```python
from build123d import *

# Parameters (mm, degrees)
SKETCH1_W               = 36
SKETCH1_H               = 36
SKETCH1_R               = 2.15
BOSS_EXTRUDE1_DEPTH     = 3
BOSS_EXTRUDE2_START     = 2
BOSS_EXTRUDE2_OUTLINE_W = 36
BOSS_EXTRUDE2_OUTLINE_H = 36
BOSS_EXTRUDE2_DEPTH     = 2


# Read off the part's stored shape, not the designer's step: Boss-Extrude2
with BuildPart() as part:
    # Sketch1 → Boss-Extrude1 (new, symmetric)
    with BuildSketch(Plane.XY):
        Rectangle(SKETCH1_W, SKETCH1_H)
        with Locations((-15.5, 15.5)):
            Circle(SKETCH1_R, mode=Mode.SUBTRACT)
        with Locations((15.5, 15.5)):
            Circle(SKETCH1_R, mode=Mode.SUBTRACT)
        with Locations((15.5, -15.5)):
            Circle(SKETCH1_R, mode=Mode.SUBTRACT)
        with Locations((-15.5, -15.5)):
            Circle(SKETCH1_R, mode=Mode.SUBTRACT)
    extrude(amount=BOSS_EXTRUDE1_DEPTH, both=True)

    # Boss-Extrude2 outline → Boss-Extrude2 (add)
    with BuildSketch(Plane.XY.offset(BOSS_EXTRUDE2_START)):
        Rectangle(BOSS_EXTRUDE2_OUTLINE_W, BOSS_EXTRUDE2_OUTLINE_H)
    extrude(amount=BOSS_EXTRUDE2_DEPTH)


solid = part.part
```
Verification items for the finished model (mm, model axes). A direction names the side the tool comes from. Give positions to 0.01 mm unless a question says otherwise; leave off trailing zeros. Order: outer loops, then holes, each group sorted by start corner. A loop starts at its lowest first (then second) coordinate and runs counter-clockwise, first axis right, second up. Notation, with made-up numbers: (-26.5, 16.25) -> (-3.5, 16.25) arc R12 ccw to (-3.5, 39.25) -> close; hole circle Ø10 at (29, 8). An arc over 180 degrees is marked (long way). One line per item, written item: value.
(1) Gauge pin test, flat ends, axial feed: pin 1 (2 mm diameter, centred on x = 16.5, y = 15, fed in from -Z); pin 2 (5 mm diameter, centred on x = 15.5, y = 15.5, fed in from -Z). Record the tip position at first contact, or that the pin passes through.
Final values:
pin 1: z = 2
pin 2: z = -3
(2) Sectioned sample at B-B on x = -15.5. Record the cut outline in (y, z), then the cut area to 3 significant figures.
Final values:
outline: (-18, -3) -> (-17.65, -3) -> (-17.65, 2) -> (-13.35, 2) -> (-13.35, -3) -> (13.35, -3) -> (13.35, 2) -> (17.65, 2) -> (17.65, -3) -> (18, -3) -> (18, 4) -> (-18, 4) -> close
area: 209 mm^2
(3) Tool access check on faces 1 (the face through (0, 18, 1)), 2 (the face through (-16, -15, 2)). Record the directions out of +Z, -Z, +X, -X, +Y, -Y that give a thin tool (end or side, any length) a straight path to the whole face; none if there is none.
Final values:
face 1: +Z, -Z, +X, -X, +Y
face 2: -Z
(4) Draft check along X on faces 3 (the face through (0, 0, 4)), 4 (the face through (-18, 0, 1)), 5 (the face through (-16, 16, 2)). Enter one of: pulls with the +X half, pulls with the -X half, needs draft (parallel to the pull), parting line crosses it, or undercut.
Final values:
face 3: needs draft
face 4: pulls with the -X half
face 5: undercut
(5) Scan lines: line 1 along Y through (x, z) = (15.5, 0); line 2 along X through (y, z) = (14, -1). Record each from-to range of solid material in increasing order. Write a range as [from, to].
Final values:
line 1: [-18, -17.65], [-13.35, 13.35], [17.65, 18]
line 2: [-18, -17.04], [-13.96, 13.96], [17.04, 18]
(6) Sectioned sample at A-A on z = 1. Record the cut outline in (x, y), then the cut area to 3 significant figures.
Final values:
outline: (-18, -18) -> (18, -18) -> (18, 18) -> (-18, 18) -> close; hole circle Ø4.3 at (-15.5, -15.5); hole circle Ø4.3 at (-15.5, 15.5); hole circle Ø4.3 at (15.5, -15.5); hole circle Ø4.3 at (15.5, 15.5)
area: 1,240 mm^2
